from build123d import *

# Parameters (mm, degrees)
SKETCH1_W      = 16
SKETCH1_H      = 16
EXTRUDE1_DEPTH = 96
SKETCH2_W      = 13
SKETCH2_H      = 13
EXTRUDE2_DEPTH = 99.630624048
SKETCH3_R      = 4
SKETCH3_R_2    = 1.85
EXTRUDE3_DEPTH = 99.630624048
SKETCH4_R      = 4
SKETCH4_R_2    = 1.85
EXTRUDE4_DEPTH = 99.630624048
FILLET1_R      = 1


with BuildPart() as part:
    # Sketch1 → Extrude1 (new body)
    with BuildSketch(Plane.XY):
        with Locations((8, 8)):
            Rectangle(SKETCH1_W, SKETCH1_H)
    extrude(amount=-EXTRUDE1_DEPTH)

    # Sketch2 → Extrude2 (cut, through all)
    with BuildSketch(Plane.XY):
        with Locations((8, 8)):
            Rectangle(SKETCH2_W, SKETCH2_H)
    extrude(amount=-EXTRUDE2_DEPTH, mode=Mode.SUBTRACT)

    # Sketch3 → Extrude3 (cut, through all)
    with BuildSketch(Plane(origin=(0, 16, 0), x_dir=(1, 0, 0), z_dir=(0, 1, 0))):
        with Locations(Location((8, 64, 0), (0, 0, 270))):
            Circle(SKETCH3_R)
        with Locations(Location((8, 32, 0), (0, 0, 270))):
            Circle(SKETCH3_R)
        with Locations((8, 0)):
            Circle(SKETCH3_R)
        with Locations((8, 96)):
            Circle(SKETCH3_R)
        with Locations((8, 128)):
            Circle(SKETCH3_R)
        with Locations((8, 160)):
            Circle(SKETCH3_R)
        with Locations((8, 192)):
            Circle(SKETCH3_R)
        with Locations((8, 224)):
            Circle(SKETCH3_R)
        with Locations((8, 256)):
            Circle(SKETCH3_R)
        with Locations(Location((8, 48, 0), (0, 0, 270))):
            Circle(SKETCH3_R)
        with Locations(Location((8, 56, 0), (0, 0, 270))):
            Circle(SKETCH3_R_2)
        with Locations(Location((8, 40, 0), (0, 0, 270))):
            Circle(SKETCH3_R_2)
        with Locations(Location((8, 80, 0), (0, 0, 270))):
            Circle(SKETCH3_R)
        with Locations(Location((8, 88, 0), (0, 0, 270))):
            Circle(SKETCH3_R_2)
        with Locations(Location((8, 72, 0), (0, 0, 270))):
            Circle(SKETCH3_R_2)
        with Locations(Location((8, 16, 0), (0, 0, 270))):
            Circle(SKETCH3_R)
        with Locations(Location((8, 24, 0), (0, 0, 270))):
            Circle(SKETCH3_R_2)
        with Locations(Location((8, 8, 0), (0, 0, 270))):
            Circle(SKETCH3_R_2)
        with Locations((8, 112)):
            Circle(SKETCH3_R)
        with Locations((8, 120)):
            Circle(SKETCH3_R_2)
        with Locations((8, 104)):
            Circle(SKETCH3_R_2)
        with Locations((8, 144)):
            Circle(SKETCH3_R)
        with Locations((8, 152)):
            Circle(SKETCH3_R_2)
        with Locations((8, 136)):
            Circle(SKETCH3_R_2)
        with Locations((8, 176)):
            Circle(SKETCH3_R)
        with Locations((8, 184)):
            Circle(SKETCH3_R_2)
        with Locations((8, 168)):
            Circle(SKETCH3_R_2)
        with Locations((8, 208)):
            Circle(SKETCH3_R)
        with Locations((8, 216)):
            Circle(SKETCH3_R_2)
        with Locations((8, 200)):
            Circle(SKETCH3_R_2)
        with Locations((8, 240)):
            Circle(SKETCH3_R)
        with Locations((8, 248)):
            Circle(SKETCH3_R_2)
        with Locations((8, 232)):
            Circle(SKETCH3_R_2)
    extrude(amount=-EXTRUDE3_DEPTH, mode=Mode.SUBTRACT)

    # Sketch4 → Extrude4 (cut, through all)
    with BuildSketch(Plane(origin=(16, 0, 0), x_dir=(0, 0, -1), z_dir=(1, 0, 0))):
        with Locations(Location((32, 8, 0), (0, 0, 90))):
            Circle(SKETCH4_R)
        with Locations(Location((64, 8, 0), (0, 0, 90))):
            Circle(SKETCH4_R)
        with Locations((0, 8)):
            Circle(SKETCH4_R)
        with Locations((96, 8)):
            Circle(SKETCH4_R)
        with Locations((128, 8)):
            Circle(SKETCH4_R)
        with Locations((160, 8)):
            Circle(SKETCH4_R)
        with Locations((192, 8)):
            Circle(SKETCH4_R)
        with Locations((224, 8)):
            Circle(SKETCH4_R)
        with Locations((256, 8)):
            Circle(SKETCH4_R)
        with Locations(Location((48, 8.074203, 0), (0, 0, 90))):
            Circle(SKETCH4_R)
        with Locations(Location((40, 8.074203, 0), (0, 0, 90))):
            Circle(SKETCH4_R_2)
        with Locations(Location((56, 8.074203, 0), (0, 0, 90))):
            Circle(SKETCH4_R_2)
        with Locations(Location((80, 8, 0), (0, 0, 90))):
            Circle(SKETCH4_R)
        with Locations(Location((72, 8, 0), (0, 0, 90))):
            Circle(SKETCH4_R_2)
        with Locations(Location((88, 8, 0), (0, 0, 90))):
            Circle(SKETCH4_R_2)
        with Locations(Location((16, 8, 0), (0, 0, 90))):
            Circle(SKETCH4_R)
        with Locations(Location((8, 8, 0), (0, 0, 90))):
            Circle(SKETCH4_R_2)
        with Locations(Location((24, 8, 0), (0, 0, 90))):
            Circle(SKETCH4_R_2)
        with Locations((112, 8)):
            Circle(SKETCH4_R)
        with Locations((104, 8)):
            Circle(SKETCH4_R_2)
        with Locations((120, 8)):
            Circle(SKETCH4_R_2)
        with Locations((144, 8)):
            Circle(SKETCH4_R)
        with Locations((136, 8)):
            Circle(SKETCH4_R_2)
        with Locations((152, 8)):
            Circle(SKETCH4_R_2)
        with Locations((176, 8)):
            Circle(SKETCH4_R)
        with Locations((168, 8)):
            Circle(SKETCH4_R_2)
        with Locations((184, 8)):
            Circle(SKETCH4_R_2)
        with Locations((208, 8)):
            Circle(SKETCH4_R)
        with Locations((200, 8)):
            Circle(SKETCH4_R_2)
        with Locations((216, 8)):
            Circle(SKETCH4_R_2)
        with Locations((240, 8)):
            Circle(SKETCH4_R)
        with Locations((232, 8)):
            Circle(SKETCH4_R_2)
        with Locations((248, 8)):
            Circle(SKETCH4_R_2)
    extrude(amount=-EXTRUDE4_DEPTH, mode=Mode.SUBTRACT)

    # Fillet1
    fillet1_edges = [part.edges().sort_by_distance(p)[0] for p in [
        (0, 16, -48),
        (16, 16, -48),
        (16, 0, -48),
        (0, 0, -48),
    ]]
    fillet(fillet1_edges, radius=FILLET1_R)


solid = part.part
Work out the finished part from the listing and answer in its coordinate system (mm). A direction names the side the tool comes from. Give positions to 0.01 mm unless a question says otherwise; leave off trailing zeros. Write each loop counter-clockwise with the first axis right and the second up, starting at its lowest first coordinate (ties: lowest second). Pieces come first, ordered by that corner, then holes.
Q1. Straight lines are drawn through the part: L1, parallel to Y at x = 11.5, z = -3.5; L2, parallel to X at y = 1.25, z = -8. For each, find the intervals that lie inside material, in ascending order.
Answer:
L1: y = 0 to 1.5, 14.5 to 16
L2: x = 0 to 6.15, 9.85 to 16
Q2. The part is cut by section C-C on z = -45. Give the vertices of the cut face in (x, y).
Answer:
outline: (0, 1) arc R1 ccw to (1, 0) - (5.35, 0) - (5.35, 1.5) - (1.5, 1.5) - (1.5, 5.43) - (0, 5.43) - close; (0, 10.72) - (1.5, 10.72) - (1.5, 14.5) - (5.35, 14.5) - (5.35, 16) - (1, 16) arc R1 ccw to (0, 15) - close; (10.65, 0) - (15, 0) arc R1 ccw to (16, 1) - (16, 5.43) - (14.5, 5.43) - (14.5, 1.5) - (10.65, 1.5) - close; (10.65, 14.5) - (14.5, 14.5) - (14.5, 10.72) - (16, 10.72) - (16, 15) arc R1 ccw to (15, 16) - (10.65, 16) - close
Q3. A tool of negligible diameter and unlimited length cuts with its end or side. For faces 1 (the face through (5.6, 0.8, -19.2)), 2 (the face through (12.2, 14.5, -47.3)), from which of +Z, -Z, +X, -X, +Y, -Y can it reach the whole face along a straight path? Write none if from no direction.
Answer:
face 1: +Y, -Y
face 2: +Z, -Z
Q4. Given pin 1 (1.5 mm diameter, centred on x = 10.5, y = 2, fed in from +Z); pin 2 (5 mm diameter, centred on x = 8, z = -56, fed in from -Y), each flat-ended and moving along its own axis, determine where each tip first touches the part or whether it passes through.
Answer:
pin 1: stops at z = -2.58
pin 2: stops at y = 0
Q5. The part is cut by section A-A on x = 3. Give the vertices of the cut face in (y, z), and give its area (3 significant figures).
Answer:
outline: (0, -96) - (1.5, -96) - (1.5, 0) - (0, 0) - close; (14.5, -96) - (16, -96) - (16, 0) - (14.5, 0) - close
area: 288 mm2
Q6. For a pull along Y with two mould halves and no side action, classify faces 3 (the face through (1, 8, -92)), 4 (the face through (5.6, 0.8, -35.2)), 5 (the face through (12.2, 1.5, -47.3)) as released by +Y, released by -Y, zero draft, split by the parting line, or undercut.
Answer:
face 3: undercut
face 4: zero draft
face 5: undercut
Q7. The part is cut by section B-B on z = -64. Give the vertices of the cut face in (x, y), and give its area (3 significant figures).
Answer:
outline: (0, 1) arc R1 ccw to (1, 0) - (4, 0) - (4, 1.5) - (1.5, 1.5) - (1.5, 4) - (0, 4) - close; (0, 12) - (1.5, 12) - (1.5, 14.5) - (4, 14.5) - (4, 16) - (1, 16) arc R1 ccw to (0, 15) - close; (12, 0) - (15, 0) arc R1 ccw to (16, 1) - (16, 4) - (14.5, 4) - (14.5, 1.5) - (12, 1.5) - close; (12, 14.5) - (14.5, 14.5) - (14.5, 12) - (16, 12) - (16, 15) arc R1 ccw to (15, 16) - (12, 16) - close
area: 38.1 mm2
